Autodesk Inventor part; units mm, degrees
ref_plane "YZ Plane" through (0, 0, 0) normal (1, 0, 0) x (0, 1, 0)
ref_plane "XZ Plane" through (0, 0, 0) normal (0, 1, 0) x (-1, 0, 0)
ref_plane "XY Plane" through (0, 0, 0) normal (0, 0, 1) x (1, 0, 0)
sketch "Sketch1" plane through (0, 0, 0) normal (0, 1, 0) x (-1, 0, 0)
  ellipse E0 centre (0, 0) end of major axis (0, 17.78) minor radius 11.2075
  line L0 (11.1609, 1.6196) -> (-11.1609, 1.6196)
  line L1 (0, -17.78) -> (0, 1.6196)
  line L2 (8.595, 11.4106) -> (-8.6719, 11.4106)
  dimension "d0" = 17.78
  dimension "d11" = 9.7909
revolve "Revolution1" add sketch "Sketch1" angle 360 about axis through (0, 0, -17.78) along (0, 0, 1) picked at (-2.3015, -10.0552) contours L0 L1 E0
sketch "Sketch2" plane through (0, 0, 1.6196) normal (0, 0, 1) x (1, 0, 0)
  line L0 (-8.636, 1.778) -> (8.636, 1.778)
  line L1 (8.636, 1.778) -> (8.636, -1.778)
  line L2 (8.636, -1.778) -> (-8.636, -1.778)
  line L3 (-8.636, -1.778) -> (-8.636, 1.778)
  line L4 (-8.636, 1.778) -> (8.636, -1.778) construction
  line L5 (8.636, 1.778) -> (-8.636, -1.778) construction
  point P0 (0, 0)
  dimension "d2" = 17.272
  dimension "d3" = 3.556
extrude "Extrusion1" cut sketch "Sketch2" against normal blind 10.16
sketch "Sketch3" plane through (0, 0, 1.6196) normal (0, 0, 1) x (1, 0, 0)
  line L0 (-5.11, 8.0772) -> (5.05, 8.0772)
  line L1 (5.05, 8.0772) -> (5.05, 5.5372)
  line L2 (5.05, 5.5372) -> (-5.11, 5.5372)
  line L3 (-5.11, 5.5372) -> (-5.11, 8.0772)
  line L4 (-5.11, 8.0772) -> (5.05, 5.5372) construction
  line L5 (5.05, 8.0772) -> (-5.11, 5.5372) construction
  circle A0 centre (0, 0) radius 11.1609
  line L6 (-11.1609, 0) -> (11.1609, 0)
  line L7 (11.2075, 0) -> (0, 0)
  line L8 (-5.11, -8.0772) -> (5.05, -8.0772)
  line L9 (5.05, -8.0772) -> (5.05, -5.5372)
  line L10 (5.05, -5.5372) -> (-5.11, -5.5372)
  line L11 (-5.11, -5.5372) -> (-5.11, -8.0772)
  point P0 (-0.03, 6.8072)
  dimension "d6" = 10.16
  dimension "d7" = 2.54
  dimension "d12" = 6.8072
extrude "Extrusion2" cut sketch "Sketch3" against normal blind 7.62 contours L0 L1 L2 L3 | L11 L10 L9 L8
sketch "Sketch4" plane through (0, 0, 1.6196) normal (0, 0, 1) x (1, 0, 0)
  circle A0 centre (0, 3.497) radius 0.889
  point P0 (0, 0)
  dimension "d13" = 1.778
extrude "Extrusion3" cut sketch "Sketch4" against normal through all
properties part number "Bead Round Top copy 1"
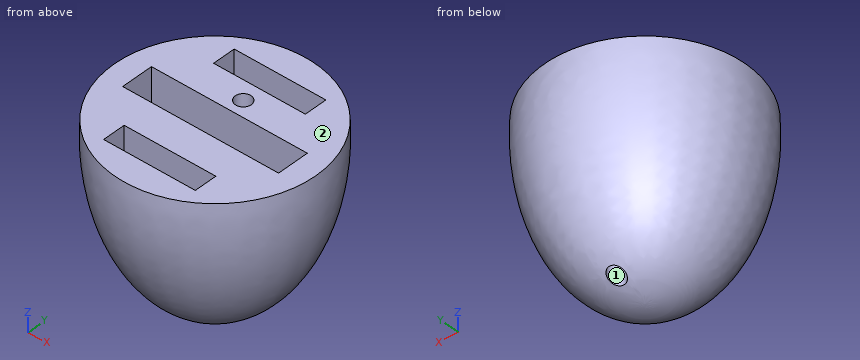
Build history of the part. All positions in model axes, mm. Face numbers are marked on the shaded views. Give positions to 0.01 mm unless a question says otherwise; leave off trailing zeros. Write item = value, one per line. Start each with the question number.
(1) Two-plate mould, pull along X, no slides. Class the marked faces 1 and 2: released by +X, released by -X, zero draft, split by the parting line, or undercut.
(2) Slice it at A-A on z = -3. State how many separate pieces and enclosed holes the cut face has, plus the area to 3 significant figures.
(3) Probe L1, parallel to Y at x = 3, z = -4.5; L2, parallel to Y at x = -0.25, z = -1.75; L3, parallel to Y at x = 4.5, z = -3.5. List the from-to ranges inside material, lowest first. Write a range as [from, to].
(4) Pin check, flat tips, straight feed: pin 1 Ø1.1 at (y, z) = (0.5, -5.5) entering from -X; pin 2 Ø8.5 at (x, z) = (1, -3.5) entering from -Y; pin 3 Ø1.8 at (x, y) = (2, -0.5) entering from +Z; pin 4 Ø4 at (y, z) = (0.5, -5.5) entering from +X. Stop position of each tip, or through.
Responses:
q1.face_1 = undercut
q1.face_2 = zero draft
q2.separate_pieces = 1
q2.enclosed_holes = 4
q2.area = 268 mm2
q3.L1 = [-10.42, -8.08], [-5.54, -1.78], [1.78, 5.54], [8.08, 10.42]
q3.L2 = [-11.15, -8.08], [-5.54, -1.78], [1.78, 2.64], [4.35, 5.54], [8.08, 11.15]
q3.L3 = [-10.02, -8.08], [-5.54, -1.78], [1.78, 5.54], [8.08, 10.02]
q4.pin_1 = -10.76
q4.pin_2 = -11.21
q4.pin_3 = -8.54
q4.pin_4 = 10.98
